Answer from the drawing. Dimensions are ordinates in mm from the lowest x, y and z of the part. Give positions to 0.01 mm unless a question says otherwise; leave off trailing zeros. Loops run counter-clockwise (first coordinate to the right, second up) from the corner with the lowest first, then second, coordinate; pieces in that order, holes last.
(1) Each of these flat-tipped pins is pushed along its axis until it touches: P1, Ø10, axis at x = 36, y = 28.5, coming from the -Z side; P2, Ø3, axis at x = 16.69, y = 37.69, coming from the +Z side. Where does it stop, or does it pass through?
(2) Find section C-C, the plane x = 28. Write down the section's boundary in (y, z), then the cut area to 3 significant figures.
(3) Straight lines are drawn through the part: probe 1 along Y at (x, z) = (51, 1); probe 2 along Y at (x, z) = (4.5, 1.75) (1 decimal); probe 3 along Y at (x, z) = (28, 1.1). For each, find the intervals that lie inside material, in ascending order.
(4) Find section B-B, the plane x = 51. Write down the section's boundary in (y, z).
(5) Find section A-A, the plane y = 6. Write down the section's boundary in (x, z), then the cut area to 3 significant figures.
(6) Find section D-D, the plane y = 49. Write down the section's boundary in (x, z), then the cut area to 3 significant figures.
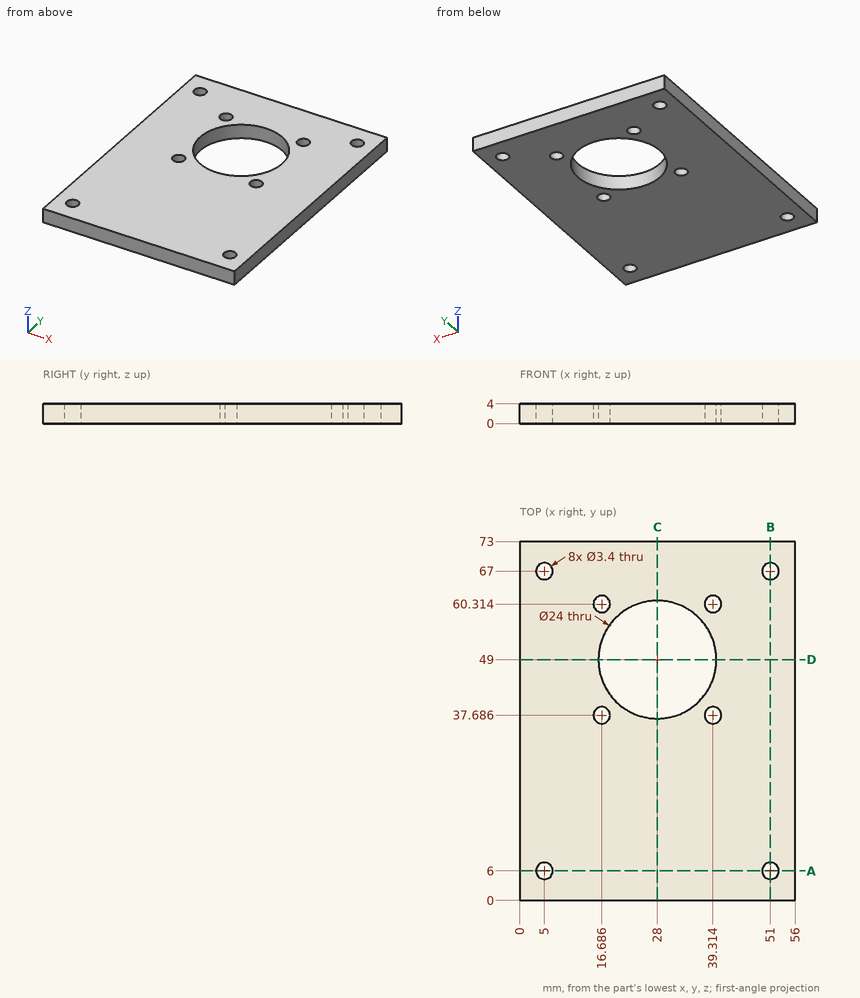
Entries:
1. P1: stops at z = 0
1. P2: passes through
2. outline: (0, 0) - (37, 0) - (37, 4) - (0, 4) - close; (61, 0) - (73, 0) - (73, 4) - (61, 4) - close
2. area: 196 mm2
3. probe 1: y = 0 to 4.3, 7.7 to 65.3, 68.7 to 73
3. probe 2: y = 0 to 4.4, 7.6 to 65.4, 68.6 to 73
3. probe 3: y = 0 to 37, 61 to 73
4. outline: (0, 0) - (4.3, 0) - (4.3, 4) - (0, 4) - close; (7.7, 0) - (65.3, 0) - (65.3, 4) - (7.7, 4) - close; (68.7, 0) - (73, 0) - (73, 4) - (68.7, 4) - close
5. outline: (0, 0) - (3.3, 0) - (3.3, 4) - (0, 4) - close; (6.7, 0) - (49.3, 0) - (49.3, 4) - (6.7, 4) - close; (52.7, 0) - (56, 0) - (56, 4) - (52.7, 4) - close
5. area: 197 mm2
6. outline: (0, 0) - (16, 0) - (16, 4) - (0, 4) - close; (40, 0) - (56, 0) - (56, 4) - (40, 4) - close
6. area: 128 mm2
